Check sheet for the modelled part. Datum: model origin and axes. Units: mm. Face numbers are marked on the shaded views. A direction names the side the tool comes from. Give positions to 0.01 mm unless a question says otherwise; leave off trailing zeros. Loops run counter-clockwise (first coordinate to the right, second up) from the corner with the lowest first, then second, coordinate; pieces in that order, holes last. Notation, with made-up numbers: (8.25, -26) -> (64.25, -26) arc R22 ccw to (64.25, -20) -> close; hole circle Ø5 at (36, -19.5). An arc over 180 degrees is marked (long way). Answer as CSV lines item,"result". Start each with the question number.
(1) Section check B-B on y = -11. Enter the section's corners in (x, z), plus the area to 3 significant figures.
(2) Release check for a two-part mould opening along Y. For the marked faces 1, 2 and 3 record: pulls with the +Y half, pulls with the -Y half, needs draft (parallel to the pull), parting line crosses it, or undercut.
(3) Section check D-D on y = 14. Enter the section's corners in (x, z), plus the area to 3 significant figures.
(4) Section check C-C on x = -319.5. Enter the section's corners in (y, z).
(5) Access from +Z, -Z, +X, -X, +Y, -Y to the whole of each face (thin tool, end or side, straight path). Record for the marked faces 4, 5 and 6.
(6) Section check A-A on z = 17.5. Enter the section's corners in (x, y).
(7) Gauge pin test, flat ends, axial feed: pin 1 Ø6 at (x, z) = (-246, -0.5) entering from -Y; pin 2 Ø1.2 at (x, y) = (-207, 79.5) entering from +Z; pin 3 Ø6 at (x, z) = (-88, -7) entering from -Y. Record the tip position at first contact, or that the pin passes through.
(8) Material ranges on line 1 (Y direction, x = -147, z = 16); line 2 (Z direction, x = -55, y = 21.5); line 3 (Z direction, x = -291.5, y = -17), recorded low to high. Write a range as from..to.
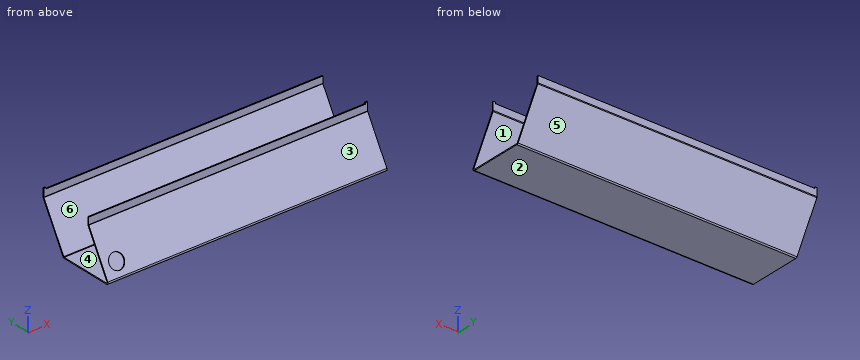
from build123d import *

# Parameters (mm, degrees)
SM_BASE_FLANGE_1_DEPTH = 400
SKETCH_7_W             = 3
SKETCH_7_H             = 1.5
EXTRUDE_1_DEPTH        = 2
SKETCH_9_R             = 10.75
CUT_EXTRUDE_2_DEPTH    = 10


# Sheet-metal steps are written as plain solids
with BuildPart() as part:
    # Sketch 1 → Базовая кромка1 (new body)
    with BuildSketch(Plane(origin=(0, 0, 0), x_dir=(0, 0, -1), z_dir=(1, 0, 0))):
        with BuildLine():
            Line((-22.356799498, 0), (-12.62474869, 0))
            ThreePointArc((-12.62474869, 0), (-12.365929645, -0.034074174), (-12.12474869, -0.133974596))
            Line((-12.12474869, -0.133974596), (45.893200502, -33.63065318))
            ThreePointArc((45.893200502, -33.63065318), (48.393200502, -33.63065318), (49.643200502, -31.465589671))
            Line((49.643200502, -31.465589671), (49.643200502, 42.760907637))
            ThreePointArc((49.643200502, 42.760907637), (49.308264012, 44.010907637), (48.393200502, 44.925971147))
            Line((48.393200502, 44.925971147), (-11.776672479, 79.665063509))
            ThreePointArc((-11.776672479, 79.665063509), (-12.379624866, 79.914814566), (-13.026672479, 80))
            Line((-13.026672479, 80), (-22.356799498, 80))
            Line((-22.356799498, 80), (-22.356799498, 78.5))
            Line((-22.356799498, 78.5), (-13.026672479, 78.5))
            ThreePointArc((-13.026672479, 78.5), (-12.767853434, 78.465925826), (-12.526672479, 78.366025404))
            Line((-12.526672479, 78.366025404), (47.643200502, 43.626933041))
            ThreePointArc((47.643200502, 43.626933041), (48.009225906, 43.260907637), (48.143200502, 42.760907637))
            Line((48.143200502, 42.760907637), (48.143200502, -31.465589671))
            ThreePointArc((48.143200502, -31.465589671), (47.643200502, -32.331615075), (46.643200502, -32.331615075))
            Line((46.643200502, -32.331615075), (-11.37474869, 1.165063509))
            ThreePointArc((-11.37474869, 1.165063509), (-11.977701077, 1.414814566), (-12.62474869, 1.5))
            Line((-12.62474869, 1.5), (-22.356799498, 1.5))
            Line((-22.356799498, 1.5), (-22.356799498, 0))
        make_face()
    extrude(amount=-SM_BASE_FLANGE_1_DEPTH)

    # Эскиз7 → Бобышка-Вытянуть1 (add)
    with BuildSketch(Plane.XY.offset(22.356799498)):
        with Locations((-398.5, 79.25)):
            Rectangle(SKETCH_7_W, SKETCH_7_H)
        with Locations((-1.5, 0.75)):
            Rectangle(SKETCH_7_W, SKETCH_7_H)
    extrude(amount=EXTRUDE_1_DEPTH)

    # Эскиз9 → Вырез-Вытянуть2 (cut)
    with BuildSketch(Plane(origin=(0, -5.350651137, 3.089199874), x_dir=(1, 0, 0), z_dir=(0, -0.86602540378444, 0.49999999999999756))):
        with Locations(Location((-380, -38.560004086, 0), (0, 0, 270))):
            Circle(SKETCH_9_R)
    extrude(amount=-CUT_EXTRUDE_2_DEPTH, mode=Mode.SUBTRACT)


solid = part.part
Working result:
1,outline,"(-400, -49.64) -> (0, -49.64) -> (0, -48.14) -> (-400, -48.14) -> close; (-400, -9.7) -> (0, -9.7) -> (0, -6.7) -> (-400, -6.7) -> close"
1,area,"1,800 mm^2"
2,face 1,"undercut"
2,face 2,"needs draft"
2,face 3,"pulls with the -Y half"
3,outline,"(-400, -49.64) -> (0, -49.64) -> (0, -48.14) -> (-400, -48.14) -> close"
3,area,"600 mm^2"
4,outline,"(-33.63, -45.89) arc R2.5 ccw to (-31.47, -49.64) -> (42.76, -49.64) arc R2.5 ccw to (44.93, -48.39) -> (79.67, 11.78) arc R2.5 ccw to (80, 13.03) -> (80, 22.36) -> (78.5, 22.36) -> (78.5, 13.03) arc R1 cw to (78.37, 12.53) -> (43.63, -47.64) arc R1 cw to (42.76, -48.14) -> (-31.47, -48.14) arc R1 cw to (-32.33, -46.64) -> (1.17, 11.37) arc R2.5 ccw to (1.5, 12.62) -> (1.5, 22.36) -> (0, 22.36) -> (0, 12.62) arc R1 cw to (-0.13, 12.12) -> close"
5,face 4,"+X, -X"
5,face 5,"-Z, +X, -X, +Y"
5,face 6,"+Z, +X, -X"
6,outline,"(-400, 0) -> (0, 0) -> (0, 1.5) -> (-400, 1.5) -> close; (-400, 78.5) -> (0, 78.5) -> (0, 80) -> (-400, 80) -> close"
7,pin 1,"stops at y = -9.15"
7,pin 2,"stops at z = 22.36"
7,pin 3,"stops at y = -12.91"
8,line 1,"y = 0..1.5, 78.5..80"
8,line 2,"z = -49.64..-48.14"
8,line 3,"z = -49.64..-48.14, -20.09..-17.09"
